Could you check a few things on this model? Use its own coordinates, in mm. A direction names the side the tool comes from. Coordinates: 2 decimals unless noted, no trailing zeros. Write each loop counter-clockwise with the first axis right and the second up, starting at its lowest first coordinate (ties: lowest second). Pieces come first, ordered by that corner, then holes. Notation, with made-up numbers: (-28, 59.5) - (-5, 59.5) arc R17 cw to (-5, 91.5) - close; hole circle Ø11 at (27.5, 9). An arc over 180 degrees is marked (long way). Answer as a JSON object with one key per item and string values. Group by question number.
1) If we section it at B-B (z = 0): Write out the boundary of the cut face in (x, y), plus the area to 3 significant figures.
2) If we section it at A-A (y = -0.5): Write out the boundary of the cut face in (x, z).
3) If we section it at C-C (y = -4.5): Write out the boundary of the cut face in (x, z).
4) Will this pin go through, and if not, where does the flat tip stop? pin 1 Ø1.5 at (x, y) = (-1, -6.5) entering from -Z.
5) Please list where these lines run through material, in increasing order: line 1 along X through (y, z) = (-1, 0.9); line 2 along Z through (x, y) = (1.3, -4.75); line 3 along Z through (x, y) = (-0.05, -1.25).
6) On a 3-axis mill with a long thin cutter (end or side, diameter ignored), from which of +Z, -Z, +X, -X, +Y, -Y can I reach the whole of each face in a straight line? I mean faces 1 (the conical face through (0.7, -7.4, 0.2)), 2 (the flat face through (0.75, -1, 0)). Say none if no direction works.
7) We'd pull the mould along X, two halves only. Please class faces 3 (the flat face through (-0.75, -1, 0)), 4 (the flat face through (1, 0, 0)), 5 (the cylindrical face through (-0.45, -3.11, -1.43)): released by +X, released by -X, zero draft, split by the parting line, or undercut.
```python
from build123d import *

# Parameters (mm, degrees)
CUT_EXTRUDE1_DEPTH = 2


with BuildPart() as part:
    # Sketch1 → Base-Revolve (revolve)
    with BuildSketch(Plane.XY, mode=Mode.PRIVATE) as base_revolve_sk:
        Polygon((0, -8), (0.4, -8), (1.5, -6), (1.5, -0.3), (1.2, 0), (0, 0), align=None)
    revolve(base_revolve_sk.sketch.rotate(Axis((0, -34, 0), (0, 1, 0)), 90), axis=Axis((0, -34, 0), (0, 1, 0)))

    # Sketch2 → Cut-Extrude1 (cut)
    with BuildSketch(Plane(origin=(0, 0, 0), x_dir=(1, 0, 0), z_dir=(0, 1, 0))):
        Polygon((0.75, 0.433012702), (0, 0.866025404), (-0.75, 0.433012702), (-0.75, -0.433012702), (0, -0.866025404), (0.75, -0.433012702), align=None)
    extrude(amount=-CUT_EXTRUDE1_DEPTH, mode=Mode.SUBTRACT)


solid = part.part
```
Here are the results:
{
 "1": {"outline": "(-1.5, -6) - (-0.4, -8) - (0.4, -8) - (1.5, -6) - (1.5, -0.3) - (1.2, 0) - (0.75, 0) - (0.75, -2) - (-0.75, -2) - (-0.75, 0) - (-1.2, 0) - (-1.5, -0.3) - close", "area": "18.7 mm²"},
 "2": {"outline": "circle Ø3 at (0, 0); hole (-0.75, -0.43) - (0, -0.87) - (0.75, -0.43) - (0.75, 0.43) - (0, 0.87) - (-0.75, 0.43) - close"},
 "3": {"outline": "circle Ø3 at (0, 0)"},
 "4": {"pin 1": "stops at z = -1.43"},
 "5": {"line 1": "x = -1.2 to 1.2", "line 2": "z = -0.75 to 0.75", "line 3": "z = -1.5 to -0.84, 0.84 to 1.5"},
 "6": {"face 1": "-Y", "face 2": "+Y"},
 "7": {"face 3": "undercut", "face 4": "zero draft", "face 5": "split by the parting line"}
}
